from build123d import *

# Parameters (mm, degrees)
F0_R     = 23.7453835504
F0_R_2   = 13.3203594212
F1_DEPTH = 6.35
F2_DEPTH = 9.525
F0_R_3   = 9.525
F3_DEPTH = 8.255
F4_DEPTH = 9.525
F5_DEPTH = 9.525


# Not quite as in the source:
# - a feature names something its author has since deleted; it is built from what else it names


with BuildPart() as f1:
    # F0 (on Front) → F1 (new body, symmetric)
    with BuildSketch(Plane.XZ):
        Circle(F0_R)
        Circle(F0_R_2, mode=Mode.SUBTRACT)
    extrude(amount=F1_DEPTH, both=True)

    # F0 (on Front) → F2 (join, symmetric)
    with BuildSketch(Plane.XZ):
        with BuildLine():
            ThreePointArc((25.9205484169, 0), (18.7722391675, 17.8739437974), (1.27, 25.8894173405))
            ThreePointArc((1.27, 25.8894173405), (0, 25.9205484169), (-1.27, 25.8894173405))
            ThreePointArc((-1.27, 25.8894173405), (-17.8739437974, -18.7722391675), (25.9205484169, 0))
        make_face()
        Circle(F0_R, mode=Mode.SUBTRACT)
    extrude(amount=F2_DEPTH, both=True)

    # F0 (on Front) → F3 (join, symmetric)
    with BuildSketch(Plane.XZ):
        Circle(F0_R_2)
        Circle(F0_R_3, mode=Mode.SUBTRACT)
    extrude(amount=F3_DEPTH, both=True)

    # F0 (on Front) → F4 (join, symmetric)
    with BuildSketch(Plane.XZ):
        with BuildLine():
            Line((1.27, 25.8894173405), (2.2161464291, 28.48893329))
            ThreePointArc((2.2161464291, 28.48893329), (0, 28.575), (-2.2161464291, 28.48893329))
            Line((-2.2161464291, 28.48893329), (-1.27, 25.8894173405))
            ThreePointArc((-1.27, 25.8894173405), (0, 25.9205484169), (1.27, 25.8894173405))
        make_face()
        with BuildLine():
            ThreePointArc((-2.2161464291, 28.48893329), (-19.406239213, -20.9744726896), (28.575, 0))
            ThreePointArc((28.575, 0), (20.9744726896, 19.406239213), (2.2161464291, 28.48893329))
            Line((2.2161464291, 28.48893329), (1.27, 25.8894173405))
            ThreePointArc((1.27, 25.8894173405), (18.7722391675, 17.8739437974), (25.9205484169, 0))
            ThreePointArc((25.9205484169, 0), (-17.8739437974, -18.7722391675), (-1.27, 25.8894173405))
            Line((-1.27, 25.8894173405), (-2.2161464291, 28.48893329))
        make_face()
    extrude(amount=F4_DEPTH, both=True)

    # F0 (on Front) → F5 (cut, symmetric)
    with BuildSketch(Plane.XZ):
        with BuildLine():
            Line((1.27, 25.8894173405), (2.2161464291, 28.48893329))
            ThreePointArc((2.2161464291, 28.48893329), (0, 28.575), (-2.2161464291, 28.48893329))
            Line((-2.2161464291, 28.48893329), (-1.27, 25.8894173405))
            ThreePointArc((-1.27, 25.8894173405), (0, 25.9205484169), (1.27, 25.8894173405))
        make_face()
    extrude(amount=F5_DEPTH, both=True, mode=Mode.SUBTRACT)


solid = f1.part
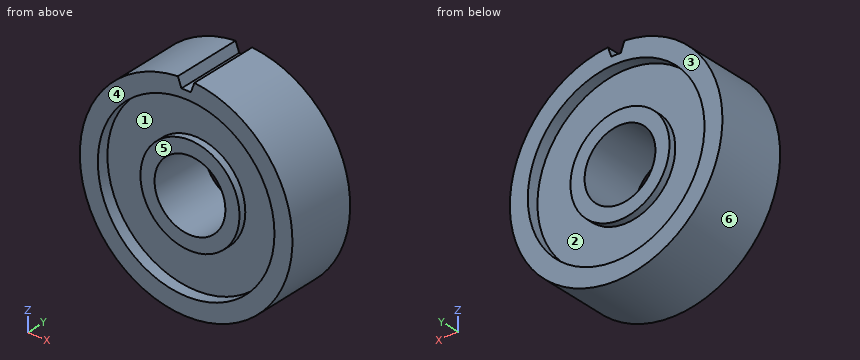
Part model, mm, in its own coordinate system. Face numbers are marked on the shaded views. A direction names the side the tool comes from. Give positions to 0.01 mm unless a question says otherwise; leave off trailing zeros. Loops run counter-clockwise (first coordinate to the right, second up) from the corner with the lowest first, then second, coordinate; pieces in that order, holes last. Notation, with made-up numbers: M -5.75,10.5 L 37.25,10.5 A22 ccw 37.25,22.5 Z; hole C 72.25,36.25 d8. An arc over 180 degrees is marked long. Put each result on its own line as item: value. Start each with the question number.
1) Saw through at A-A (z = 0). List the corners of the cut face in (x, y) (3 decimals).
2) Pull direction Z, two halves, no side cores. Call the marked faces 4, 5 and 6: +Z half, -Z half, draft (parallel to the pull), parting line (faces both ways), or undercut.
3) Saw through at D-D (x = 19.5). List the corners of the cut face in (y, z) (3 decimals), then the cut area to 3 significant figures.
4) Probe probe 1 along Z at (x, y) = (0, -7.7) (3 decimals); probe 2 along X at (y, z) = (-7.75, 4); probe 3 along Z at (x, y) = (-3, -6.75). List the from-to ranges inside material, lowest first.
5) 3-axis set-ups, long thin cutter, end or side, ignore diameter. For the marked faces 1, 2 and 3: which of +Z, -Z, +X, -X, +Y, -Y reach the whole face in a straight line?
6) Saw through at C-C (z = 10.5). List the corners of the cut face in (x, y) (3 decimals), then the cut area to 3 significant figures.
7) Flat gauge pins, fed straight in: pin 1 (14 mm diameter, centred on x = -8, z = 5.5, fed in from -Y) (3 decimals); pin 2 (8 mm diameter, centred on x = 6, z = -1, fed in from +Y) (3 decimals); pin 3 (8 mm diameter, centred on y = -2, z = 8.5, fed in from +X); pin 4 (17 mm diameter, centred on x = 0, z = 0, fed in from +Y). Where does each tip first touch, or does it go through?
8) Saw through at B-B (x = 0). List the corners of the cut face in (y, z) (3 decimals), then the cut area to 3 significant figures.
Numbers:
1. outline: M -28.575,-9.525 L -23.745,-9.525 L -23.745,-6.35 L -13.32,-6.35 L -13.32,-8.255 L -9.525,-8.255 L -9.525,8.255 L -13.32,8.255 L -13.32,6.35 L -23.745,6.35 L -23.745,9.525 L -28.575,9.525 Z; M 9.525,-8.255 L 13.32,-8.255 L 13.32,-6.35 L 23.745,-6.35 L 23.745,-9.525 L 28.575,-9.525 L 28.575,9.525 L 23.745,9.525 L 23.745,6.35 L 13.32,6.35 L 13.32,8.255 L 9.525,8.255 Z
2. face 4: draft
2. face 5: undercut
2. face 6: parting line
3. outline: M -9.525,-20.887 L 9.525,-20.887 L 9.525,-13.55 L 6.35,-13.55 L 6.35,13.55 L 9.525,13.55 L 9.525,20.887 L -9.525,20.887 L -9.525,13.55 L -6.35,13.55 L -6.35,-13.55 L -9.525,-13.55 Z
3. area: 624 mm^2
4. probe 1: -28.575 to -23.745, -13.32 to -9.525, 9.525 to 13.32, 23.745 to 25.921
4. probe 2: -28.29 to -23.41, -12.71 to -8.64, 8.64 to 12.71, 23.41 to 28.29
4. probe 3: -28.42 to -23.56, -12.98 to -9.04, 9.04 to 12.98, 23.56 to 28.42
5. face 1: -Y
5. face 2: +Y
5. face 3: +Z, -Z, +X, -X, +Y
6. outline: M -26.576,-9.525 L -21.298,-9.525 L -21.298,-6.35 L -8.196,-6.35 L -8.196,-8.255 L 8.196,-8.255 L 8.196,-6.35 L 21.298,-6.35 L 21.298,-9.525 L 26.576,-9.525 L 26.576,9.525 L 21.298,9.525 L 21.298,6.35 L 8.196,6.35 L 8.196,8.255 L -8.196,8.255 L -8.196,6.35 L -21.298,6.35 L -21.298,9.525 L -26.576,9.525 Z
6. area: 805 mm^2
7. pin 1: y = -8.255
7. pin 2: y = 8.255
7. pin 3: x = 28.22
7. pin 4: through
8. outline: M -9.525,-28.575 L 9.525,-28.575 L 9.525,-23.745 L 6.35,-23.745 L 6.35,-13.32 L 8.255,-13.32 L 8.255,-9.525 L -8.255,-9.525 L -8.255,-13.32 L -6.35,-13.32 L -6.35,-23.745 L -9.525,-23.745 Z; M -9.525,23.745 L -6.35,23.745 L -6.35,13.32 L -8.255,13.32 L -8.255,9.525 L 8.255,9.525 L 8.255,13.32 L 6.35,13.32 L 6.35,23.745 L 9.525,23.745 L 9.525,25.921 L -9.525,25.921 Z
8. area: 524 mm^2
